from build123d import *

# Parameters (mm, degrees)
SKETCH2_R           = 30.5
SKETCH2_R_2         = 28.5
BOSS_EXTRUDE2_DEPTH = 1
SKETCH7_R           = 36.5
SKETCH7_R_2         = 30.5
SKETCH7_R_3         = 34.9
BOSS_EXTRUDE3_DEPTH = 7
SKETCH7_3_R         = 36.5
SKETCH7_3_R_2       = 34.9
BOSS_EXTRUDE5_DEPTH = 8
SKETCH14_R          = 1.85
CUT_EXTRUDE1_DEPTH  = 8
CIRPATTERN1_COUNT   = 3
SWEEP1_OUTLINE_R    = 30.5
SWEEP1_OUTLINE_R_2  = 28.5
SWEEP1_ANGLE        = 90


# Read off the part's stored shape, not the designer's step: Sweep1
with BuildPart() as part:
    # Sketch2 → Boss-Extrude2 (new body)
    with BuildSketch(Plane(origin=(0, 50, 0), x_dir=(1, 0, 0), z_dir=(0, 1, 0))):
        with Locations(Location((0, 0, 0), (0, 0, 270))):
            Circle(SKETCH2_R)
        with Locations(Location((0, 0, 0), (0, 0, 270))):
            Circle(SKETCH2_R_2, mode=Mode.SUBTRACT)
    extrude(amount=BOSS_EXTRUDE2_DEPTH)



with BuildPart() as body_2:
    # Sketch7 → Boss-Extrude3 (new body)
    # profile 1 of 2: a face of its own
    with BuildSketch(Plane(origin=(0, 51, 0), x_dir=(1, 0, 0), z_dir=(0, 1, 0))):
        with Locations(Location((0, 0, 0), (0, 0, 270))):
            Circle(SKETCH7_R)
        with Locations(Location((0, 0, 0), (0, 0, 270))):
            Circle(SKETCH7_R_2, mode=Mode.SUBTRACT)
    # profile 2 of 2: a face of its own
    with BuildSketch(Plane(origin=(0, 51, 0), x_dir=(1, 0, 0), z_dir=(0, 1, 0))):
        with Locations(Location((0, 0, 0), (0, 0, 270))):
            Circle(SKETCH7_R)
        Circle(SKETCH7_R_3, mode=Mode.SUBTRACT)
    extrude(amount=-BOSS_EXTRUDE3_DEPTH)


with BuildPart() as part_1:
    add(part.part)

    add(body_2.part)  # Boss-Extrude5 merges body 2
    # Sketch7<3> → Boss-Extrude5 (add)
    with BuildSketch(Plane(origin=(0, 51, 0), x_dir=(1, 0, 0), z_dir=(0, 1, 0))):
        with Locations(Location((0, 0, 0), (0, 0, 270))):
            Circle(SKETCH7_3_R)
        with Locations(Location((0, 0, 0), (0, 0, 270))):
            Circle(SKETCH7_3_R_2, mode=Mode.SUBTRACT)
    extrude(amount=BOSS_EXTRUDE5_DEPTH)

    # Sketch14 → Cut-Extrude1 (cut)
    with BuildSketch(Plane.XY.offset(36.5)):
        with Locations(Location((0, 55, 0), (0, 0, 270))):
            Circle(SKETCH14_R)
    cut_extrude1 = extrude(amount=-CUT_EXTRUDE1_DEPTH, mode=Mode.SUBTRACT)

    # CirPattern1: Cut-Extrude1 ×3 about axis
    cirpattern1_axis = Axis((0, 0, 0), (0, 1, 0))
    for i in range(1, CIRPATTERN1_COUNT):
        add(cut_extrude1.rotate(cirpattern1_axis, i * 360 / CIRPATTERN1_COUNT), mode=Mode.SUBTRACT)

    # Sweep1 outline → Sweep1 (revolve)
    with BuildSketch(Plane(origin=(0, 50, 54.842660898), x_dir=(0, -1, 0), z_dir=(0, 0, 1))):
        with Locations((54.842660898, 0)):
            Circle(SWEEP1_OUTLINE_R)
        with Locations((54.842660898, 0)):
            Circle(SWEEP1_OUTLINE_R_2, mode=Mode.SUBTRACT)
    revolve(axis=Axis((0, 50, 54.842660898), (1, 0, 0)), revolution_arc=SWEEP1_ANGLE)


solid = part_1.part
Design review of the part built by this model. Coordinates are the model's own, in mm. A direction names the side the tool comes from. Round coordinates to 2 decimals unless told otherwise and drop trailing zeros. Loops run counter-clockwise (first coordinate to the right, second up) from the corner with the lowest first, then second, coordinate; pieces in that order, holes last. Notation, with made-up numbers: (64.25, 7.5) - (71.25, 7.5) arc R30 cw to (71.25, 30.5) - close; hole circle Ø3 at (-14, 4.5). An arc over 180 degrees is marked (long way). One line per item, written item: value. Start each with the question number.
1) For faces 1 (the flat face through (0, 51, -29)), 2 (the flat face through (-8, 44, -30)), 3 (the cylindrical face through (0.08, 56.85, 35.69)), 4 (the flat face through (-30, 59, 19)), list the 3-axis set-ups (+Z, -Z, +X, -X, +Y, -Y) from which the entire face can be reached by the end or side of a thin tool; tool diameter is ignored.
2) To check wall thickness, follow L1, parallel to X at y = 50.7, z = 0; L2, parallel to X at y = 6.5, z = 21; L3, parallel to Y at x = 0, z = 35. State the ranges of each line that lie inside material, in increasing order. Write a range as from..to.
3) Consider section D-D on x = -10. Give the boundary of the cut face in (y, z).
4) Insertion check: pin 1 Ø21 at (x, z) = (8.5, 14) entering from +Y; pin 2 Ø22 at (x, z) = (-16, 0) entering from -Y; pin 3 Ø8 at (x, z) = (-0.5, 39) entering from -Y; pin 4 Ø12 at (y, z) = (44.5, 44.5) entering from +X. Each pin has a flat end and moves straight along its axis. Give the tip position at first contact, or say it passes through.
5) Consider section A-A on y = 55. Give the boundary of the cut face in (x, z), then the cut area to 3 significant figures.
6) Consider section C-C on x = 0. Give the boundary of the cut face in (y, z).
7) Consider section B-B on x = 26.5. Give the boundary of the cut face in (y, z), then the cut area to 3 significant figures.
8) Draft analysis for pull direction X (two halves, no side actions). For faces 5 (the cylindrical face through (-30.962, 54.944, 16.104)), 6 (the cylindrical face through (-35.632, 51.605, -7.912)), 7 (the cylindrical face through (-27.82, 50.49, -6.18)), 8 (the flat face through (9.2, 22.4, 54.843)), state which applies: +X half, -X half, draft (parallel to the pull), parting line (faces both ways), or undercut.
Reported:
1. face 1: +Y
1. face 2: none
1. face 3: +Z
1. face 4: +Z, -Z, +X, -X, +Y
2. L1: x = -36.5..-28.5, 28.5..36.5
2. L2: x = -30.5..-28.5, 28.5..30.5
2. L3: y = -33..-30.95, 32.67..35.9, 44..53.15, 56.85..59
3. outline: (-33.66, 54.84) arc R83.66 ccw to (50, -28.81) - (44, -28.81) - (44, -35.1) - (59, -35.1) - (59, -33.44) - (51, -33.44) - (51, -26.69) - (50, -26.69) arc R81.53 cw to (-31.53, 54.84) - close; (21.85, 54.84) arc R28.15 ccw to (50, 26.69) - (51, 26.69) - (51, 33.44) - (59, 33.44) - (59, 35.1) - (44, 35.1) - (44, 29.52) arc R26.03 cw to (23.97, 54.84) - close
4. pin 1: stops at y = -11.86
4. pin 2: stops at y = -20.12
4. pin 3: stops at y = -34.51
4. pin 4: passes through
5. outline: (-32.49, -16.62) - (-31.11, -15.82) arc R34.9 cw to (-1.85, 34.85) - (-1.85, 36.45) arc R36.5 ccw to start; (-30.64, -19.83) arc R36.5 ccw to (30.64, -19.83) - (29.26, -19.03) arc R34.9 cw to (-29.26, -19.03) - close; (1.85, 34.85) arc R34.9 cw to (31.11, -15.82) - (32.49, -16.62) arc R36.5 ccw to (1.85, 36.45) - close
5. area: 341 mm^2
6. outline: (-35.34, 54.84) arc R85.34 ccw to (50, -30.5) - (44, -30.5) - (44, -36.5) - (59, -36.5) - (59, -34.9) - (51, -34.9) - (51, -28.5) - (50, -28.5) arc R83.34 cw to (-33.34, 54.84) - close; (23.66, 54.84) arc R26.34 ccw to (50, 28.5) - (51, 28.5) - (51, 34.9) - (53.15, 34.9) - (53.15, 36.5) - (44, 36.5) - (44, 31.25) arc R24.34 cw to (25.66, 54.84) - close; (56.85, 34.9) - (59, 34.9) - (59, 36.5) - (56.85, 36.5) - close
7. outline: (-19.94, 54.84) arc R69.94 ccw to (50, -15.1) - (44, -15.1) - (44, -25.1) - (59, -25.1) - (59, -22.71) - (51, -22.71) - (51, -10.49) - (50, -10.49) arc R65.33 cw to (-15.33, 54.84) - close; (5.65, 54.84) arc R44.35 ccw to (50, 10.49) - (51, 10.49) - (51, 22.71) - (59, 22.71) - (59, 25.1) - (44, 25.1) - (44, 15.56) arc R39.74 cw to (10.26, 54.84) - close
7. area: 981 mm^2
8. face 5: undercut
8. face 6: parting line
8. face 7: undercut
8. face 8: draft
